from build123d import *

# Parameters (mm, degrees)
F0_W     = 115
F0_H     = 15
F1_DEPTH = 10
F2_W     = 15
F2_H     = 10
F3_DEPTH = 5
F4_W     = 5
F4_H     = 10
F5_DEPTH = 25
F6_W     = 10
F6_H     = 3.5
F7_DEPTH = 10


with BuildPart() as f1:
    # F0 (on Front) → F1 (new body)
    with BuildSketch(Plane.XZ):
        Rectangle(F0_W, F0_H)
    extrude(amount=F1_DEPTH)

    # F2 (on face) → F3 (cut)
    with BuildSketch(Plane.XY.offset(7.5)):
        with Locations((50, -5)):
            Rectangle(F2_W, F2_H)
    extrude(amount=-F3_DEPTH, mode=Mode.SUBTRACT)

    # F4 (on face) → F5 (join)
    with BuildSketch(Plane.XY.offset(7.5)):
        with Locations((-55, -5)):
            Rectangle(F4_W, F4_H)
    extrude(amount=F5_DEPTH)

    # F6 (on face) → F7 (join)
    with BuildSketch(Plane(origin=(-57.5, 0, 0), x_dir=(0, -1, 0), z_dir=(-1, 0, 0))):
        with Locations((5, 30.75)):
            Rectangle(F6_W, F6_H)
    extrude(amount=F7_DEPTH)


solid = f1.part
CAD build for the part. Positions are in the model's coordinates, mm. A direction names the side the tool comes from. Give positions to 0.01 mm unless a question says otherwise; leave off trailing zeros. Loops run counter-clockwise (first coordinate to the right, second up) from the corner with the lowest first, then second, coordinate; pieces in that order, holes last. Notation, with made-up numbers: M -20.75,75.25 L 9.25,75.25 A13 ccw 9.25,87.25 Z; hole C -29.75,65.5 d8. An arc over 180 degrees is marked long. Answer in a Markdown table with one row per item. Add a question column.
Item 1: Band-saw the part on C-C on x = 3.5. Give the cut face in (y, z).
Item 2: Band-saw the part on B-B on z = 19. Give the cut face in (x, y), then the cut area to 3 significant figures.
Item 3: Tool access for faces 1 (the face through (42.5, -5, 5)), 2 (the face through (-57.5, -5, 10)), 3 (the face through (-1, -5, -7.5)): list every direction of +Z, -Z, +X, -X, +Y, -Y with a clear straight run to the whole face (end or side of a thin tool).
Item 4: Drop flat-ended pins along their axis: P1, Ø5, axis at y = -2, z = 28, coming from the +X side; P2, Ø6, axis at y = -8, z = 4.5, coming from the -X side; P3, Ø3, axis at x = 9.5, z = 3.5, coming from the +Y side; P4, Ø5, axis at x = -47, y = -9, coming from the +Z side. Give the stop position or say it passes through.
Item 5: Probe probe 1 along X at (y, z) = (-6.25, -4.5); probe 2 along Z at (x, y) = (-22, -4); probe 3 along X at (y, z) = (-5.75, 3). List the from-to ranges inside material, lowest first.
Item 6: Band-saw the part on A-A on y = -8.75. Give the cut face in (x, z).
Reply:
| question | item | result |
|---|---|---|
| 1 | outline | M -10,-7.5 L 0,-7.5 L 0,7.5 L -10,7.5 Z |
| 2 | outline | M -57.5,-10 L -52.5,-10 L -52.5,0 L -57.5,0 Z |
| 2 | area | 50.0 mm^2 |
| 3 | face 1 | +Z, +X, +Y, -Y |
| 3 | face 2 | -Z, -X, +Y, -Y |
| 3 | face 3 | -Z, +X, -X, +Y, -Y |
| 4 | P1 | stops at x = -52.5 |
| 4 | P2 | stops at x = -57.5 |
| 4 | P3 | stops at y = 0 |
| 4 | P4 | stops at z = 7.5 |
| 5 | probe 1 | x = -57.5 to 57.5 |
| 5 | probe 2 | z = -7.5 to 7.5 |
| 5 | probe 3 | x = -57.5 to 42.5 |
| 6 | outline | M -67.5,29 L -57.5,29 L -57.5,-7.5 L 57.5,-7.5 L 57.5,2.5 L 42.5,2.5 L 42.5,7.5 L -52.5,7.5 L -52.5,32.5 L -67.5,32.5 Z |
